Verification items for this drawing (mm, ordinates from the low corner). Coordinates: 2 decimals unless noted, no trailing zeros. Order: outer loops, then holes, each group sorted by start corner. A loop starts at its lowest first (then second) coordinate and runs counter-clockwise, first axis right, second up.
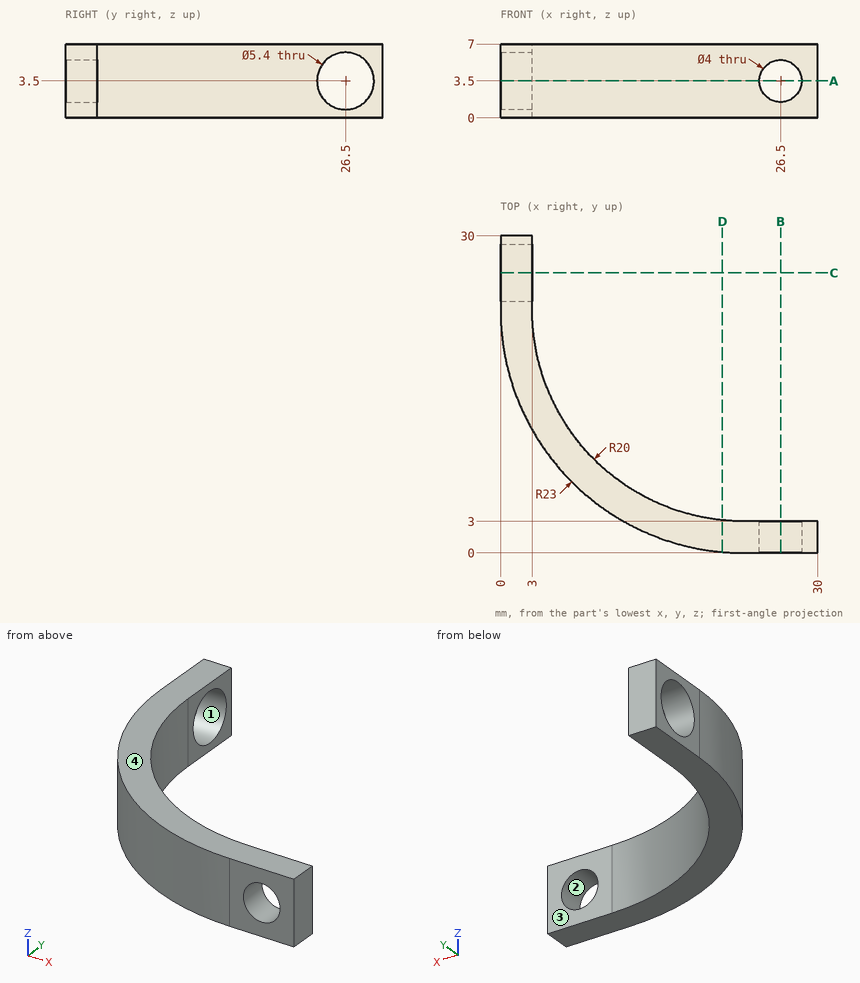
(1) Cross-section at A-A (z = 3.5). Enter the section's corners in (x, y), and give its area (3 significant figures).
Filled in:
outline: (0, 23) arc R23 ccw to (23, 0) - (24.5, 0) - (24.5, 3) - (23, 3) arc R20 cw to (3, 23) - (3, 23.8) - (0, 23.8) - close; (0, 29.2) - (3, 29.2) - (3, 30) - (0, 30) - close; (28.5, 0) - (30, 0) - (30, 3) - (28.5, 3) - close
area: 115 mm2
(2) Thickness scan on probe 1 along Z at (x, y) = (26.5, 1.05); probe 2 along Y at (x, z) = (1.85, 3.5); probe 3 along Y at (x, z) = (29.5, 2). Record the ranges inside material, lowest first.
Filled in:
probe 1: z = 0 to 1.5, 5.5 to 7
probe 2: y = 13.96 to 23.8, 29.2 to 30
probe 3: y = 0 to 3
(3) Cross-section at C-C (y = 26.5). Enter the section's corners in (x, z), and give its area (3 significant figures).
Filled in:
outline: (0, 0) - (3, 0) - (3, 0.8) - (0, 0.8) - close; (0, 6.2) - (3, 6.2) - (3, 7) - (0, 7) - close
area: 4.80 mm2
(4) Release check for a two-part mould opening along Z. For the marked faces 1, 2, 3 and 4 record: +Z half, -Z half, draft (parallel to the pull), parting line (faces both ways), or undercut.
Filled in:
face 1: undercut
face 2: undercut
face 3: draft
face 4: +Z half
(5) Cross-section at B-B (x = 26.5). Enter the section's corners in (y, z), and give its area (3 significant figures).
Filled in:
outline: (0, 0) - (3, 0) - (3, 1.5) - (0, 1.5) - close; (0, 5.5) - (3, 5.5) - (3, 7) - (0, 7) - close
area: 9.00 mm2
(6) Cross-section at D-D (x = 21). Enter the section's corners in (y, z), and give its area (3 significant figures).
Filled in:
outline: (0.09, 0) - (3.1, 0) - (3.1, 7) - (0.09, 7) - close
area: 21.1 mm2
(7) Go/stop test with flat-tipped pins: P1, Ø2, axis at y = 22, z = 2.5, coming from the +X side; P2, Ø2, axis at x = 27, z = 5, coming from the +Y side; P3, Ø4, axis at x = 9.5, z = 4.5, coming from the +Y side. Record where each tip stops, or that it passes through.
Filled in:
P1: stops at x = 3.1
P2: stops at y = 3
P3: stops at y = 10.36
